```python
from build123d import *

# Parameters (mm, degrees)
ESQUISSE1_W             = 4
ESQUISSE1_H             = 3.5
ESQUISSE2_R             = 2
BOSS_EXTRU_1_DEPTH      = 14
ENL_V_MAT_EXTRU_1_DEPTH = 2
CHANFREIN1_SIZE         = 0.39
CONG_1_R                = 0.2


with BuildPart() as part:
    # Esquisse1 → Révolution1 (revolve)
    with BuildSketch(Plane(origin=(0, 0, 0), x_dir=(-1, 0, 0), z_dir=(0, 0, -1)), mode=Mode.PRIVATE) as r_volution1_sk:
        with Locations((-2, 1.75)):
            Rectangle(ESQUISSE1_W, ESQUISSE1_H)
    revolve(r_volution1_sk.sketch.rotate(Axis((4, 0, 0), (-1, 0, 0)), 270), axis=Axis((4, 0, 0), (-1, 0, 0)))

    # Esquisse2 → Boss.-Extru.1 (add)
    with BuildSketch(Plane(origin=(4, 0, 0), x_dir=(0, 0, -1), z_dir=(1, 0, 0))):
        with Locations(Location((0, 0, 0), (0, 0, 180))):
            Circle(ESQUISSE2_R)
    extrude(amount=BOSS_EXTRU_1_DEPTH)

    # Esquisse3 → Enlèv. mat.-Extru.1 (cut)
    with BuildSketch(Plane.ZY):
        Polygon((0, -1.773042677), (1.5355, -0.886521338), (1.5355, 0.886521338), (0, 1.773042677), (-1.5355, 0.886521338), (-1.5355, -0.886521338), align=None)
    extrude(amount=-ENL_V_MAT_EXTRU_1_DEPTH, mode=Mode.SUBTRACT)

    # Esquisse4 → Enlèvement de matière-Révolution1 (revolve, cut)
    with BuildSketch(Plane.XY, mode=Mode.PRIVATE) as enl_vement_de_mati_re_r_volution1_sk:
        Polygon((2, 1.5355), (2, 0), (2.886521338, 0), align=None)
    revolve(enl_vement_de_mati_re_r_volution1_sk.sketch.rotate(Axis((2, 0, 0), (1, 0, 0)), 90), axis=Axis((2, 0, 0), (1, 0, 0)), mode=Mode.SUBTRACT)

    # Chanfrein1
    chanfrein1_edges = [part.edges().sort_by_distance(p)[0] for p in [
        (18, 0, -2),
    ]]
    chamfer(chanfrein1_edges, length=CHANFREIN1_SIZE)

    # Congé1
    cong_1_edges = [part.edges().sort_by_distance(p)[0] for p in [
        (0, 0, -3.5),
        (4, 0, -2),
    ]]
    fillet(cong_1_edges, radius=CONG_1_R)


solid = part.part
```
Input: part model. Units: mm. Frame: model coordinates. A direction names the side the tool comes from. Give positions to 0.01 mm unless a question says otherwise; leave off trailing zeros. Order: outer loops, then holes, each group sorted by start corner. A loop starts at its lowest first (then second) coordinate and runs counter-clockwise, first axis right, second up. Notation, with made-up numbers: M 34,-0.5 L 88,-0.5 A23 cw 88,22.5 Z; hole C 29.5,56 d6. An arc over 180 degrees is marked long. Return JSON: item names as keys, results as strings.
1) Line query: L1, parallel to X at y = -1.75, z = -2; L2, parallel to Y at x = 10.5, z = 0; L3, parallel to Y at x = 16.75, z = -1.5. Output: solid intervals per line, ascending. Write a range as [from, to].
Taken from the geometry:
{"L1": "x = [0, 4]", "L2": "y = [-2, 2]", "L3": "y = [-1.32, 1.32]"}
2) Section query A-A on x = 1. Output: boundary loops of the cut face in (y, z), and give its area (3 significant figures).
Taken from the geometry:
{"outline": "C 0,0 d7; hole M -1.77,0 L -0.89,-1.54 L 0.89,-1.54 L 1.77,0 L 0.89,1.54 L -0.89,1.54 Z", "area": "30.3 mm2"}
3) Mould query, pull axis Z, two halves, no side actions, for faces 1 (the face through (2.073, -3.417, -0.759)), 2 (the face through (0.986, -1.336, 0.757)), 3 (the face through (18, 0, 0)). Classes: released by +Z, released by -Z, zero draft, split by the parting line, or undercut.
Taken from the geometry:
{"face 1": "split by the parting line", "face 2": "undercut", "face 3": "zero draft"}
4) Contact query for flat-ended pins moving along their axis: pin 1 (1.5 mm diameter, centred on x = 8.5, z = -1, fed in from +Y); pin 2 (4 mm diameter, centred on x = 5.5, z = 1, fed in from +Y); pin 3 (0.5 mm diameter, centred on x = 1, y = 0.5, fed in from -Z); pin 4 (0.6 mm diameter, centred on y = 0.5, z = -1, fed in from -X). Output: stop coordinate, or through.
Taken from the geometry:
{"pin 1": "stops at y = 1.98", "pin 2": "stops at y = 3.5", "pin 3": "stops at z = -3.49", "pin 4": "stops at x = 2.07"}
5) Section query B-B on x = 15. Output: boundary loops of the cut face in (y, z).
Taken from the geometry:
{"outline": "C 0,0 d4"}
6) Access query for faces 4 (the face through (4, -2, 2)), 5 (the face through (0, 2, -1)), 6 (the face through (0.986, 1.324, 0.778)). Directions: +Z, -Z, +X, -X, +Y, -Y. A direction counts if a zero-diameter tool reaches every point of the face in a straight line with its end or side. Return the directions, or none.
Taken from the geometry:
{"face 4": "+X", "face 5": "+Z, -Z, -X, +Y, -Y", "face 6": "-X"}
